Autodesk Inventor part; units mm, degrees
ref_plane "YZ Plane" through (0, 0, 0) normal (1, 0, 0) x (0, 1, 0)
ref_plane "XZ Plane" through (0, 0, 0) normal (0, 1, 0) x (-1, 0, 0)
ref_plane "XY Plane" through (0, 0, 0) normal (0, 0, 1) x (1, 0, 0)
sketch "Esboço1" plane through (0, 0, 0) normal (1, 0, 0) x (0, 1, 0)
  circle A0 centre (0, 0) radius 49
  dimension "d0" = 98
extrude "Extrusão1" add sketch "Esboço1" along normal blind 1.5
sketch "Esboço2" plane through (1.5, 0, 0) normal (1, 0, 0) x (0, 0, -1)
  circle A0 centre (0, 0) radius 49
  circle A1 centre (0, 0) radius 47
  dimension "d3" = 2
extrude "Extrusão2" add sketch "Esboço2" along normal blind 3
sketch "Esboço3" plane through (0, 0, 0) normal (-1, 0, 0) x (0, 0, 1)
  line L0 (5, 0) -> (2.5, -4.3301)
  line L1 (2.5, -4.3301) -> (-2.5, -4.3301)
  line L2 (-2.5, -4.3301) -> (-5, 0)
  line L3 (-5, 0) -> (-2.5, 4.3301)
  line L4 (-2.5, 4.3301) -> (2.5, 4.3301)
  line L5 (2.5, 4.3301) -> (5, 0)
  point P0 (0, 0)
  point P1 (0, 0)
  dimension "d6" = 10
extrude "Extrusão3" add sketch "Esboço3" along normal blind 3
properties part number "Base"
Model file for the job. Use its own axes, mm. A direction names the side the tool comes from. Give positions to 0.01 mm unless a question says otherwise; leave off trailing zeros. Write each loop counter-clockwise with the first axis right and the second up, starting at its lowest first coordinate (ties: lowest second). Pieces come first, ordered by that corner, then holes. Notation, with made-up numbers: (34, 39) -> (58, 39) arc R14 cw to (58, 48) -> close; hole circle Ø8 at (47, 87.25). An arc over 180 degrees is marked (long way). Use CSV: the item, a comma, the result in double quotes. Start each with the question number.
1) Tool access for faces 4 (the flat face through (-1.48, -2.2, -3.73)), 5 (the flat face through (-1.48, -2.13, 3.77)), 6 (the cylindrical face through (2.98, -14.12, -44.83)), 7 (the flat face through (-1.48, 2.13, -3.77)), 8 (the flat face through (-1, -4.33, 0)): list every direction of +Z, -Z, +X, -X, +Y, -Y with a clear straight run to the whole face (end or side of a thin tool).
2) Pin check, flat tips, straight feed: P1, Ø1.5, axis at x = -1, y = 12.5, coming from the +Z side; P2, Ø1.5, axis at x = 3.5, z = -8.5, coming from the -Y side; P3, Ø2, axis at x = 0, z = 18.5, coming from the +Y side; P4, Ø3, axis at y = -9.5, z = -26, coming from the +X side. Stop position of each tip, or through.
3) Drill centre lines: L1, parallel to Y at x = 3.3, z = 0; L2, parallel to X at y = -8, z = -5; L3, parallel to Z at x = 3.75, y = 5.5. Where is each one in solid material? Low to high.
4) Two-plate mould, pull along Z, no slides. Class faces 1 (the flat face through (-1, 4.33, 0)), 2 (the flat face through (1.5, -1, 1)), 3 (the flat face through (-1.48, 2.2, 3.73)): released by +Z, released by -Z, zero draft, split by the parting line, or undercut.
5) Cut at C-C on x = -1.5. List the corners of the cut face in (y, z).
6) Cut at B-B on z = -9. List the corners of the cut face in (x, y).
7) Cut at A-A on y = -21. List the corners of the cut face in (x, z).
8) Cut at D-D on y = 3. List the corners of the cut face in (x, z), plus the area to 3 significant figures.
Final values:
1,face 4,"-Z, -X, -Y"
1,face 5,"+Z, -X, -Y"
1,face 6,"+X"
1,face 7,"-Z, -X, +Y"
1,face 8,"+Z, -Z, -X, -Y"
2,P1,"passes through"
2,P2,"stops at y = -48.38"
2,P3,"stops at y = 45.77"
2,P4,"stops at x = 1.5"
3,L1,"y = -49 to -47, 47 to 49"
3,L2,"x = 0 to 1.5"
3,L3,"z = -48.69 to -46.68, 46.68 to 48.69"
4,face 1,"zero draft"
4,face 2,"undercut"
4,face 3,"released by +Z"
5,outline,"(-4.33, -2.5) -> (0, -5) -> (4.33, -2.5) -> (4.33, 2.5) -> (0, 5) -> (-4.33, 2.5) -> close"
6,outline,"(0, -48.17) -> (4.5, -48.17) -> (4.5, -46.13) -> (1.5, -46.13) -> (1.5, 46.13) -> (4.5, 46.13) -> (4.5, 48.17) -> (0, 48.17) -> close"
7,outline,"(0, -44.27) -> (4.5, -44.27) -> (4.5, -42.05) -> (1.5, -42.05) -> (1.5, 42.05) -> (4.5, 42.05) -> (4.5, 44.27) -> (0, 44.27) -> close"
8,outline,"(-3, -3.27) -> (0, -3.27) -> (0, -48.91) -> (4.5, -48.91) -> (4.5, -46.9) -> (1.5, -46.9) -> (1.5, 46.9) -> (4.5, 46.9) -> (4.5, 48.91) -> (0, 48.91) -> (0, 3.27) -> (-3, 3.27) -> close"
8,area,"178 mm2"
